Read the model definition and answer for the solid it produces. Units are mm, in the model's axes. Face numbers are marked on the shaded views. A direction names the side the tool comes from. Give positions to 0.01 mm unless a question says otherwise; leave off trailing zeros. Loops run counter-clockwise (first coordinate to the right, second up) from the corner with the lowest first, then second, coordinate; pieces in that order, holes last. Notation, with made-up numbers: (-0.5, -39.5) -> (41.5, -39.5) arc R16 cw to (41.5, -27.5) -> close; hole circle Ø1 at (10, 19). An arc over 180 degrees is marked (long way). Write each question's results on one line, items separated by ' | '. Start each with the question number.
Item 1: Each of these flat-tipped pins is pushed along its axis until it touches: P1, Ø1.5, axis at y = -7.5, z = 3.5, coming from the +X side; P2, Ø6, axis at x = 2, y = -9.5, coming from the +Z side; P3, Ø1.6, axis at y = 30.5, z = 3, coming from the -X side; P4, Ø1.5, axis at x = -6, z = 2, coming from the +Y side. Where does it stop, or does it pass through?
Item 2: Determine the mould class of the marked faces 1, 2 and 3 for opening direction X: +X half, -X half, draft (parallel to the pull), parting line (faces both ways), or undercut.
Item 3: Which of the six approach directions +Z, -Z, +X, -X, +Y, -Y give full straight-line access (tool end or side, diameter ignored) to the marked faces 4, 5, 6 and 7?
Item 4: Section C-C on x = -5 is taken. Write down the section's boundary in (y, z).
Item 5: Section D-D on y = -12.5 is taken. Write down the section's boundary in (x, z), and give its area (3 significant figures).
Item 6: Find the intervals of material crossed by line 1 (Y direction, x = -0.5, z = 1.9); line 2 (Y direction, x = 13.5, z = 0.8); line 3 (X direction, y = -12, z = 4.1), in increasing order.
Item 7: Section A-A on y = 19 is taken. Write down the section's boundary in (x, z).
Item 8: Section B-B on x = -20 is taken. Write down the section's boundary in (y, z).
```python
from build123d import *

# Parameters (mm, degrees)
F1_DEPTH = 5
F3_DEPTH = 5


with BuildPart() as f1:
    # F0 (on Top) → F1 (new body)
    with BuildSketch(Plane.XY):
        Polygon((-3.879217, 4.916668), (-3.927753, 6.405906), (-3.844433, 6.405906), (-3.844433, 22.24392), (-3.800751, 24.223369), (-3.466664, 25.280638), (-2.567135, 25.706135), (-0.81176, 25.786219), (6.433814, 25.786219), (11.910261, 25.061419), (15.364386, 23.003504), (17.155354, 20.150413), (18.823365, 15.84125), (20.727583, 15.318682), (22.194171, 16.179382), (21.842287, 20.738504), (21.474225, 24.951404), (21.170876, 28.300369), (21.013135, 30.249078), (19.420355, 30.143108), (16.641685, 30.064642), (12.990181, 30.016107), (8.795077, 29.999119), (-10.501916, 29.999119), (-23.646198, 30.249078), (-24.396884, 28.620705), (-23.8185, 27.049765), (-21.539748, 26.629122), (-19.078178, 25.970654), (-17.677922, 24.639967), (-17.050194, 21.902552), (-16.905395, 17.021477), (-16.905395, -16.850793), (-17.050194, -21.761799), (-17.677922, -24.487888), (-19.078178, -25.773276), (-21.539748, -26.37431), (-25.835968, -27.050574), (-26.407071, -28.648208), (-25.835968, -30.249078), (-17.084978, -30.060598), (-10.163784, -29.999928), (1.632822, -29.999928), (13.100195, -30.060598), (22.615623, -30.249078), (23.690689, -27.603072), (24.857973, -23.811624), (25.848911, -19.597915), (26.407071, -15.674611), (25.840821, -15.0032), (24.874961, -14.669112), (23.831443, -14.735444), (23.037075, -15.253159), (21.241253, -18.654704), (19.547356, -21.235186), (17.870447, -23.099767), (16.132869, -24.37302), (14.258581, -25.162535), (12.165882, -25.583987), (9.782779, -25.751435), (7.026759, -25.786219), (2.927108, -25.64142), (0.241465, -25.202172), (-1.440297, -24.469283), (-2.497567, -23.424956), (-3.625214, -20.063048), (-3.927753, -14.744343), (-3.927753, -3.878004), (-3.879217, -2.301402), (-3.581532, -1.47225), (-2.826801, -1.14787), (-1.399851, -1.095289), (4.920309, -1.095289), (7.829216, -1.266782), (9.707548, -1.977022), (10.874832, -3.509133), (11.661111, -6.151093), (12.082563, -8.424992), (13.859779, -9.012274), (15.453369, -8.340863), (15.197747, 1.265164), (15.453369, 10.867956), (13.859779, 11.513482), (12.082563, 10.95613), (11.661111, 8.678187), (10.874832, 6.088806), (9.707548, 4.58339), (7.829216, 3.88124), (4.920309, 3.705702), (-1.399851, 3.705702), (-2.826801, 3.776888), (-3.581532, 4.110166), align=None)
    extrude(amount=F1_DEPTH)

    # F2 (on Top) → F3 (join)
    with BuildSketch(Plane.XY):
        with BuildLine():
            ThreePointArc((-2.816698, 31.999119), (-1.316698, 33.499119), (0.183302, 31.999119))
            Line((0.183302, 31.999119), (1.183302, 31.999119))
            ThreePointArc((1.183302, 31.999119), (-1.316698, 34.499119), (-3.816698, 31.999119))
            Line((-3.816698, 31.999119), (-2.816698, 31.999119))
        make_face()
        with BuildLine():
            Line((1.183302, 31.999119), (0.183302, 31.999119))
            ThreePointArc((0.183302, 31.999119), (-1.316698, 30.499119), (-2.816698, 31.999119))
            Line((-2.816698, 31.999119), (-3.816698, 31.999119))
            Line((-3.816698, 31.999119), (-3.816698, 29.999119))
            Line((-3.816698, 29.999119), (1.183302, 29.999119))
            Line((1.183302, 29.999119), (1.183302, 31.999119))
        make_face()
    extrude(amount=F3_DEPTH)


solid = f1.part
```
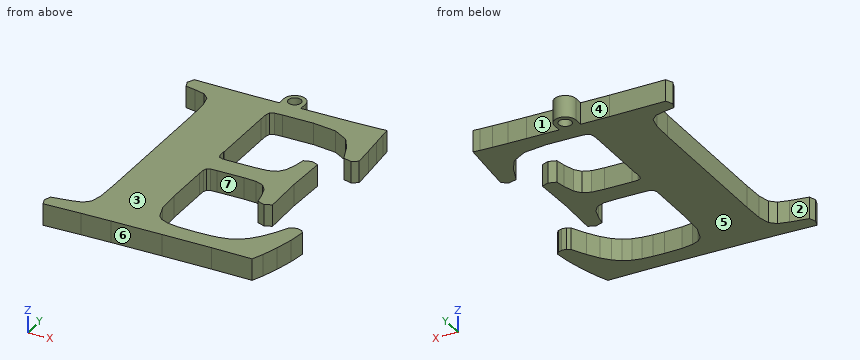
Findings:
1) P1: x = 15.45 | P2: through | P3: x = -23.9 | P4: y = 30
2) face 1: undercut | face 2: -X half | face 3: draft
3) face 4: +Z, -Z, +Y | face 5: -Z, +X, -X, +Y, -Y | face 6: +Z, -Z, -Y | face 7: +Z, -Z
4) outline: (-30, 0) -> (30, 0) -> (30, 5) -> (-30, 5) -> close
5) outline: (-16.91, 0) -> (-3.93, 0) -> (-3.93, 5) -> (-16.91, 5) -> close | area: 64.9 mm2
6) line 1: -30 to -24.88, -1.1 to 3.71, 25.79 to 30.74, 33.26 to 34.36 | line 2: -30.07 to -25.32, -8.89 to 11.4, 24.11 to 30.02 | line 3: -16.91 to -3.93
7) outline: (-16.96, 0) -> (-3.84, 0) -> (-3.84, 5) -> (-16.96, 5) -> close; (17.6, 0) -> (21.98, 0) -> (21.98, 5) -> (17.6, 5) -> close
8) outline: (-30.12, 0) -> (-26, 0) -> (-26, 5) -> (-30.12, 5) -> close; (26.22, 0) -> (30.18, 0) -> (30.18, 5) -> (26.22, 5) -> close
